Source: CAD feature listing. Evaluate the final solid. Frame: model axes, mm. Give positions to 0.01 mm unless a question says otherwise; leave off trailing zeros. Write each loop counter-clockwise with the first axis right and the second up, starting at its lowest first coordinate (ties: lowest second). Pieces come first, ordered by that corner, then holes. Notation, with made-up numbers: (3, 20) -> (16, 20) arc R21 ccw to (16, 38) -> close; hole circle Ø2 at (56.5, 66). An arc over 180 degrees is marked (long way). Use one line per item in the form item = value. Start each with the question number.
(1) Cut plane B-B, the plane z = 5.75. Output: boundary loops of the cut face in (x, y), and give its area (3 significant figures).
(2) Cut plane D-D, the plane x = 115.5. Output: boundary loops of the cut face in (y, z), and give its area (3 significant figures).
(3) Material intervals for line 1 along Y through (x, z) = (292, 5.5); line 2 along Y through (x, z) = (400, 7.5); line 3 along X through (y, z) = (-9, 1.5), sorted ascending. Write a range as from..to.
(4) Cut plane A-A, the plane x = 432. Output: boundary loops of the cut face in (y, z), and give its area (3 significant figures).
(5) Cut plane C-C, the plane y = 0. Output: boundary loops of the cut face in (x, z).
(6) First-contact query: P1, Ø6, axis at y = -35, z = 5.5, coming from the -X side; P2, Ø6, axis at x = 235.5, z = 3, coming from the -Y side; P3, Ø12, axis at x = 432, y = 0, coming from the +Z side; P4, Ø4, axis at x = 66.44, y = -11.3, coming from the -Z side. Flat tips, straight axial feed; report the tip coordinate or a pass-through.
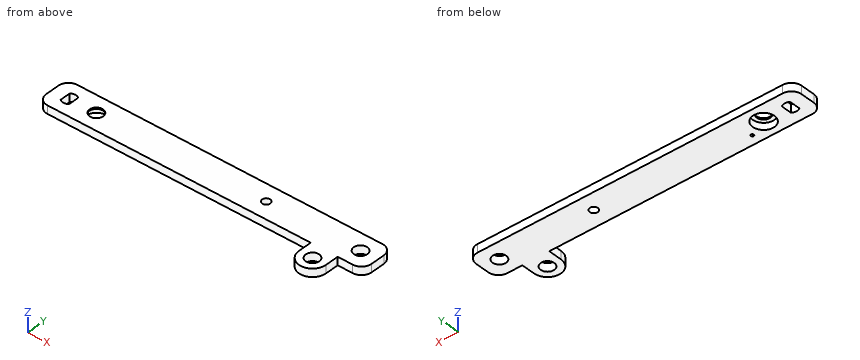
from build123d import *

# Parameters (mm, degrees)
CROQUIS1_R              = 10
CROQUIS1_R_2            = 6
SALIENTE_EXTRUIR1_DEPTH = 12
CROQUIS2_R              = 2.144956207
CORTAR_EXTRUIR1_DEPTH   = 3
CROQUIS3_R              = 16
CORTAR_EXTRUIR2_DEPTH   = 10
REDONDEO1_R             = 15
REDONDEO2_R             = 15


with BuildPart() as part:
    # Croquis1 → Saliente-Extruir1 (new body)
    with BuildSketch(Plane.XY):
        with BuildLine():
            Line((380, -45.4), (380, -25.4))
            Line((380, -25.4), (-25.4, -25.4))
            Line((-25.4, -25.4), (-25.4, 25.4))
            Line((-25.4, 25.4), (457.4, 25.4))
            Line((457.4, 25.4), (457.4, -25.4))
            Line((457.4, -25.4), (420, -25.4))
            Line((420, -25.4), (420, -45.4))
            ThreePointArc((420, -45.4), (400, -65.4), (380, -45.4))
        make_face()
        with Locations((432, 0)):
            Circle(CROQUIS1_R, mode=Mode.SUBTRACT)
        with Locations((40, 0)):
            Circle(CROQUIS1_R, mode=Mode.SUBTRACT)
        with Locations((292, 0)):
            Circle(CROQUIS1_R_2, mode=Mode.SUBTRACT)
        with Locations((400, -45.4)):
            Circle(CROQUIS1_R, mode=Mode.SUBTRACT)
        with BuildLine():
            Line((-6.28, -7.782133384), (-6.28, 7.782133384))
            ThreePointArc((-6.28, 7.782133384), (0, 10), (6.28, 7.782133384))
            Line((6.28, 7.782133384), (6.28, -7.782133384))
            ThreePointArc((6.28, -7.782133384), (0, -10), (-6.28, -7.782133384))
        make_face(mode=Mode.SUBTRACT)
    extrude(amount=SALIENTE_EXTRUIR1_DEPTH)

    # Croquis2 → Cortar-Extruir1 (cut)
    with BuildSketch(Plane(origin=(0, 0, 0), x_dir=(-1, 0, 0), z_dir=(0, 0, -1))):
        with Locations((-66.437001332, -11.298220954)):
            Circle(CROQUIS2_R)
    extrude(amount=-CORTAR_EXTRUIR1_DEPTH, mode=Mode.SUBTRACT)

    # Croquis3 → Cortar-Extruir2 (cut)
    with BuildSketch(Plane(origin=(0, 0, 0), x_dir=(-1, 0, 0), z_dir=(0, 0, -1))):
        with Locations((-40, 0)):
            Circle(CROQUIS3_R)
    extrude(amount=-CORTAR_EXTRUIR2_DEPTH, mode=Mode.SUBTRACT)

    # Redondeo1
    redondeo1_edges = [part.edges().sort_by_distance(p)[0] for p in [
        (-25.4, 25.4, 6),
        (-25.4, -25.4, 6),
    ]]
    fillet(redondeo1_edges, radius=REDONDEO1_R)

    # Redondeo2
    redondeo2_edges = [part.edges().sort_by_distance(p)[0] for p in [
        (457.4, 25.4, 6),
        (457.4, -25.4, 6),
    ]]
    fillet(redondeo2_edges, radius=REDONDEO2_R)


solid = part.part
Geometry says:
q1.outline = (-25.4, -10.4) arc R15 ccw to (-10.4, -25.4) -> (380, -25.4) -> (380, -45.4) arc R20 ccw to (420, -45.4) -> (420, -25.4) -> (442.4, -25.4) arc R15 ccw to (457.4, -10.4) -> (457.4, 10.4) arc R15 ccw to (442.4, 25.4) -> (-10.4, 25.4) arc R15 ccw to (-25.4, 10.4) -> close; hole (-6.28, -7.78) arc R10 ccw to (6.28, -7.78) -> (6.28, 7.78) arc R10 ccw to (-6.28, 7.78) -> close; hole circle Ø32 at (40, 0); hole circle Ø12 at (292, 0); hole circle Ø20 at (400, -45.4); hole circle Ø20 at (432, 0)
q1.area = 24,000 mm^2
q2.outline = (-25.4, 0) -> (25.4, 0) -> (25.4, 12) -> (-25.4, 12) -> close
q2.area = 610 mm^2
q3.line_1 = -25.4..-6, 6..25.4
q3.line_2 = -65.4..-55.4, -35.4..25.4
q3.line_3 = -25.4..-4.36, 4.36..26.77, 53.23..427.64, 436.36..457.4
q4.outline = (-25.4, 0) -> (-10, 0) -> (-10, 12) -> (-25.4, 12) -> close; (10, 0) -> (25.4, 0) -> (25.4, 12) -> (10, 12) -> close
q4.area = 370 mm^2
q5.outline = (-25.4, 0) -> (-6.28, 0) -> (-6.28, 12) -> (-25.4, 12) -> close; (6.28, 0) -> (24, 0) -> (24, 10) -> (30, 10) -> (30, 12) -> (6.28, 12) -> close; (50, 10) -> (56, 10) -> (56, 0) -> (286, 0) -> (286, 12) -> (50, 12) -> close; (298, 0) -> (422, 0) -> (422, 12) -> (298, 12) -> close; (442, 0) -> (457.4, 0) -> (457.4, 12) -> (442, 12) -> close
q6.P1 = 380
q6.P2 = -25.4
q6.P3 = through
q6.P4 = 3
